Read the model definition and answer for the solid it produces. Units are mm, in the model's axes. A direction names the side the tool comes from. Coordinates: 2 decimals unless noted, no trailing zeros. Loops run counter-clockwise (first coordinate to the right, second up) from the corner with the lowest first, then second, coordinate; pieces in that order, holes last. Notation, with made-up numbers: (37, 30.5) -> (95, 30.5) arc R25 cw to (95, 69.5) -> close; hole circle Ø4 at (67, 13). An arc over 180 degrees is marked (long way). Answer as CSV lines item,"result".
```python
from build123d import *

# Parameters (mm, degrees)
F1_DEPTH = 2
F2_DEPTH = 8.7
F3_W     = 36
F3_H     = 8.7
F4_DEPTH = 2
F5_DEPTH = 2
F6_DEPTH = 2
F7_DEPTH = 2
F8_W     = 16
F8_H     = 8.7
F9_DEPTH = 2
F10_R    = 1.99999
F11_R    = 1.99999


# Not quite as in the source:
# - a fillet or chamfer is up to 0.001 mm smaller than in the source, because OpenCascade refuses the exact size


with BuildPart() as f1:
    # F0 (on Top) → F1 (new body)
    with BuildSketch(Plane.XY):
        with BuildLine():
            Line((57, 29.5), (-57, 29.5))
            ThreePointArc((-57, 29.5), (-60.5355339059, 28.0355339059), (-62, 24.5))
            Line((-62, 24.5), (-62, -24.5))
            ThreePointArc((-62, -24.5), (-60.5355339059, -28.0355339059), (-57, -29.5))
            Line((-57, -29.5), (57, -29.5))
            ThreePointArc((57, -29.5), (60.5355339059, -28.0355339059), (62, -24.5))
            Line((62, -24.5), (62, 24.5))
            ThreePointArc((62, 24.5), (60.5355339059, 28.0355339059), (57, 29.5))
        make_face()
        with BuildLine():
            Line((-56, 27.021933794), (-55, 27.021933794))
            ThreePointArc((-55, 27.021933794), (-51.4644660941, 25.5574677), (-50, 22.021933794))
            Line((-50, 22.021933794), (-50, 12.021933794))
            ThreePointArc((-50, 12.021933794), (-51.4644660941, 8.4863998881), (-55, 7.021933794))
            Line((-55, 7.021933794), (-56, 7.021933794))
            ThreePointArc((-56, 7.021933794), (-59.5355339059, 8.4863998881), (-61, 12.021933794))
            Line((-61, 12.021933794), (-61, 22.021933794))
            ThreePointArc((-61, 22.021933794), (-59.5355339059, 25.5574677), (-56, 27.021933794))
        make_face(mode=Mode.SUBTRACT)
    extrude(amount=F1_DEPTH)

    # F0 (on Top) → F2 (join)
    with BuildSketch(Plane.XY):
        with BuildLine():
            Line((57, 31.5), (-57, 31.5))
            ThreePointArc((-57, 31.5), (-61.9497474683, 29.4497474683), (-64, 24.5))
            Line((-64, 24.5), (-64, -24.5))
            ThreePointArc((-64, -24.5), (-61.9497474683, -29.4497474683), (-57, -31.5))
            Line((-57, -31.5), (57, -31.5))
            ThreePointArc((57, -31.5), (61.9497474683, -29.4497474683), (64, -24.5))
            Line((64, -24.5), (64, 24.5))
            ThreePointArc((64, 24.5), (61.9497474683, 29.4497474683), (57, 31.5))
        make_face()
        with BuildLine():
            ThreePointArc((-62, 24.5), (-60.5355339059, 28.0355339059), (-57, 29.5))
            Line((-57, 29.5), (57, 29.5))
            ThreePointArc((57, 29.5), (60.5355339059, 28.0355339059), (62, 24.5))
            Line((62, 24.5), (62, -24.5))
            ThreePointArc((62, -24.5), (60.5355339059, -28.0355339059), (57, -29.5))
            Line((57, -29.5), (-57, -29.5))
            ThreePointArc((-57, -29.5), (-60.5355339059, -28.0355339059), (-62, -24.5))
            Line((-62, -24.5), (-62, 24.5))
        make_face(mode=Mode.SUBTRACT)
    extrude(amount=F2_DEPTH)

    # F3 (on face) → F4 (cut)
    with BuildSketch(Plane.XZ.offset(31.5)):
        with Locations((-33.0772541165, 4.35)):
            Rectangle(F3_W, F3_H)
    extrude(amount=-F4_DEPTH, mode=Mode.SUBTRACT)

    # F5 (add): a face of the model
    f5_faces = [f1.faces().sort_by_distance(p)[0] for p in [
        (64, 0, 4.35),
    ]]
    extrude(f5_faces, amount=-F5_DEPTH)

    # F6 (add): a face of the model
    f6_faces = [f1.faces().sort_by_distance(p)[0] for p in [
        (64, 0, 4.35),
    ]]
    extrude(f6_faces, amount=-F6_DEPTH)

    # F7 (cut): a face of the model
    f7_faces = [f1.faces().sort_by_distance(p)[0] for p in [
        (64, 0, 4.35),
    ]]
    extrude(f7_faces, amount=-F7_DEPTH, mode=Mode.SUBTRACT)

    # F8 (on face) → F9 (cut)
    with BuildSketch(Plane(origin=(-64, 0, 0), x_dir=(0, -1, 0), z_dir=(-1, 0, 0))):
        with Locations((-15.7182565033, 4.35)):
            Rectangle(F8_W, F8_H)
    extrude(amount=-F9_DEPTH, mode=Mode.SUBTRACT)

    # F10 (radius 2 in the source; OpenCascade refuses exactly that, so slightly less here)
    f10_edges = [f1.edges().sort_by_distance(p)[0] for p in [
        (61.949747, 29.449747, 8.7),
        (0, 31.5, 8.7),
        (-61.949747, 29.449747, 8.7),
    ]]
    fillet(f10_edges, radius=F10_R)

    # F11 (radius 2 in the source; OpenCascade refuses exactly that, so slightly less here)
    f11_edges = [f1.edges().sort_by_distance(p)[0] for p in [
        (-64, -8.390872, 8.7),
        (-54.038627, -31.5, 8.7),
        (-61.949747, -29.449747, 8.7),
        (20.961373, -31.5, 8.7),
        (61.949747, -29.449747, 8.7),
    ]]
    fillet(f11_edges, radius=F11_R)


solid = f1.part
```
Q1. Find the intervals of material crossed by probe 1 along Y at (x, z) = (-1, 3.75); probe 2 along Z at (x, y) = (37.5, -21); probe 3 along Y at (x, z) = (42, 8), in increasing order. Write a range as [from, to].
Results:
probe 1,"y = [-31.5, -29.5], [29.5, 31.5]"
probe 2,"z = [0, 2]"
probe 3,"y = [-31.02, -29.5], [29.5, 31.02]"
Q2. For a pull along X with two mould halves and no side action, classify faces 1 (the face through (-62, -29.4, 3.3)), 2 (the face through (1, 0, 0)), 3 (the face through (-1, 29.5, 5)), 4 (the face through (62, 29.4, 3.3)) as pulls with the +X half, pulls with the -X half, needs draft (parallel to the pull), parting line crosses it, or undercut.
Results:
face 1,"pulls with the -X half"
face 2,"needs draft"
face 3,"undercut"
face 4,"pulls with the +X half"
Q3. Given pin 1 Ø0.6 at (x, z) = (63, 3.5) entering from +Y; pin 2 Ø1.5 at (x, z) = (-30, 6) entering from -Y; pin 3 Ø0.6 at (y, z) = (24, 5) entering from +X, each flat-ended and moving along its own axis, determine where each tip first touches the part or whether it passes through.
Results:
pin 1,"stops at y = 28.56"
pin 2,"stops at y = 29.5"
pin 3,"stops at x = -62"
Q4. A cutting plane is placed at B-B, the plane y = 16. Write down the section's boundary in (x, z), and give its area (3 significant figures).
Results:
outline,"(-62, 0) -> (-61, 0) -> (-61, 2) -> (-62, 2) -> close; (-50, 0) -> (62, 0) -> (62, 2) -> (-50, 2) -> close"
area,"226 mm²"
Q5. A cutting plane is placed at A-A, the plane z = 3.75. Write down the section's boundary in (x, y).
Results:
outline,"(-64, -24.5) arc R7 ccw to (-57, -31.5) -> (-51.08, -31.5) -> (-51.08, -29.5) -> (-57, -29.5) arc R5 cw to (-62, -24.5) -> (-62, 7.72) -> (-64, 7.72) -> close; (-64, 23.72) -> (-62, 23.72) -> (-62, 24.5) arc R5 cw to (-57, 29.5) -> (57, 29.5) arc R5 cw to (62, 24.5) -> (64, 24.5) arc R7 ccw to (57, 31.5) -> (-57, 31.5) arc R7 ccw to (-64, 24.5) -> close; (-15.08, -31.5) -> (57, -31.5) arc R7 ccw to (64, -24.5) -> (62, -24.5) arc R5 cw to (57, -29.5) -> (-15.08, -29.5) -> close"
Q6. For faces 5 (the face through (20, -31.5, 3)), 6 (the face through (-51.504, 25.596, 0.986)), 7 (the face through (-1, 0, 2)), determine the directions among +Z, -Z, +X, -X, +Y, -Y from which every point of the face is accessible in a straight line to the end or side of a thin tool.
Results:
face 5,"+Z, -Z, +X, -X, -Y"
face 6,"+Z, -Z"
face 7,"+Z"
